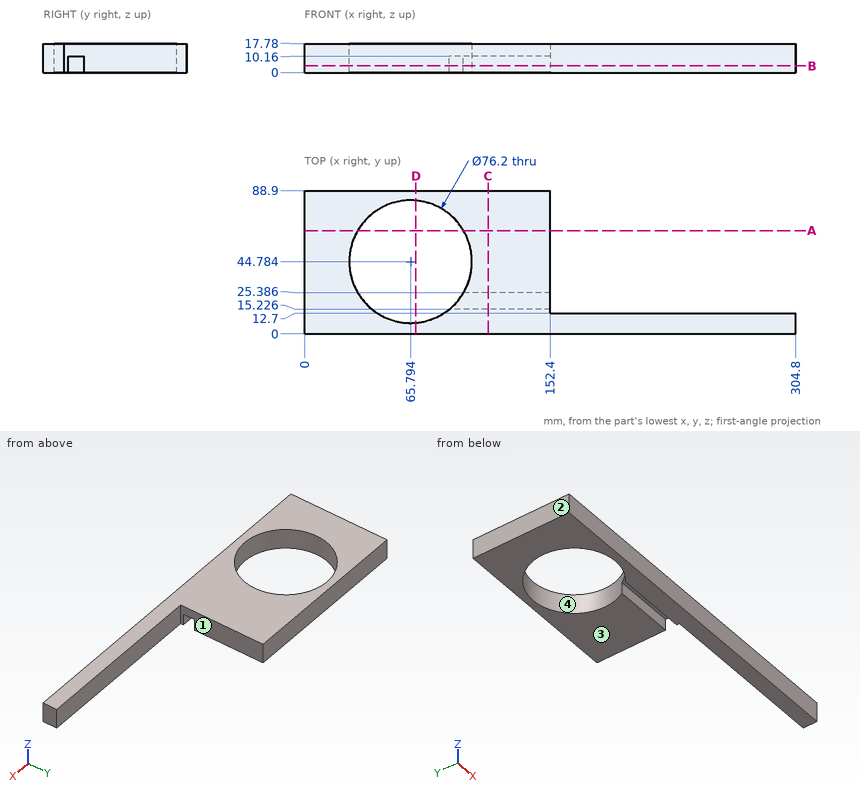
Design review of the part shown in the three views and the two pictorial views. Dimensions are in mm from the part's minimum x, y and z. A direction names the side the tool comes from. Coordinates: 2 decimals unless noted, no trailing zeros. Loops run counter-clockwise (first coordinate to the right, second up) from the corner with the lowest first, then second, coordinate; pieces in that order, holes last. Notation, with made-up numbers: M 55,-17 L 89,-17 A6 cw 89,-10 Z; hole C -39,-31 d5. An arc over 180 degrees is marked long. One line per question, with ' | ' between items.
(1) For pin 1 Ø10 at (x, z) = (77, 13.5) entering from -Y; pin 2 Ø2 at (y, z) = (62, 10) entering from +X; pin 3 Ø4 at (x, z) = (259, 15.5) entering from +Y; pin 4 Ø5 at (x, y) = (130, 22) entering from -Z, all flat-tipped, find the tip position at first contact; note any pin that passes through.
Filled in:
pin 1: stops at y = 0 | pin 2: stops at x = 152.4 | pin 3: stops at y = 12.7 | pin 4: stops at z = 10.16
(2) Wall thickness on probe 1 along Y at (x, z) = (123, 2.5); probe 2 along X at (y, z) = (43, 15.25); probe 3 along X at (y, z) = (48.5, 7.25) (1 decimal): over which ranges is each line inside the solid? List them lowest first.
Filled in:
probe 1: y = 0 to 15.23, 25.39 to 88.9 | probe 2: x = 0 to 27.74, 103.85 to 152.4 | probe 3: x = 0 to 27.9, 103.7 to 152.4
(3) We need section B-B (z = 4.25). Give the boundary of the cut face in (x, y) (1 decimal).
Filled in:
outline: M 0,0 L 304.8,0 L 304.8,12.7 L 152.4,12.7 L 152.4,15.2 L 89.8,15.2 A38.1 cw long 98.6,25.4 L 152.4,25.4 L 152.4,88.9 L 0,88.9 Z
(4) We need section A-A (y = 64). Give the boundary of the cut face in (x, z) (1 decimal), and give its area (3 significant figures).
Filled in:
outline: M 0,0 L 32.9,0 L 32.9,17.8 L 0,17.8 Z; M 98.7,0 L 152.4,0 L 152.4,17.8 L 98.7,17.8 Z | area: 1,540 mm^2
(5) We need section D-D (x = 69). Give the boundary of the cut face in (y, z), and give its area (3 significant figures).
Filled in:
outline: M 0,0 L 6.82,0 L 6.82,17.78 L 0,17.78 Z; M 82.75,0 L 88.9,0 L 88.9,17.78 L 82.75,17.78 Z | area: 231 mm^2
(6) We need section C-C (x = 114). Give the boundary of the cut face in (y, z).
Filled in:
outline: M 0,0 L 15.23,0 L 15.23,10.16 L 25.39,10.16 L 25.39,0 L 88.9,0 L 88.9,17.78 L 0,17.78 Z
(7) Draft analysis for pull direction Y (two halves, no side actions). For the marked faces 3 and 4, state which applies: released by +Y, released by -Y, zero draft, split by the parting line, or undercut.
Filled in:
face 3: zero draft | face 4: undercut
(8) Machinability: for the marked faces 1 and 2, which of the approach directions +Z, -Z, +X, -X, +Y, -Y give a long, thin tool a straight path to every point of the face, cutting with its end or side? Answer none if there is none.
Filled in:
face 1: +Z, -Z, +X, +Y | face 2: +Z, -Z, -X, +Y, -Y
